from build123d import *

# Parameters (mm, degrees)
SKETCH1_R               = 9.525
BOSS_EXTRUDE1_DEPTH     = 25.4
CUT_EXTRUDE1_DEPTH      = 29.750847814
CUT_EXTRUDE1_DEPTH_BACK = 29.750847814
SKETCH2_R               = 3.175
SKETCH3_W               = 33.02
SKETCH3_H               = 34.544
BOSS_EXTRUDE2_DEPTH     = 254
BOSS_EXTRUDE3_DEPTH     = 22.225
SKETCH5_R               = 19.05
BOSS_EXTRUDE4_DEPTH     = 76.2
SKETCH6_W               = 19.05
SKETCH6_H               = 17.78
SKETCH6_R               = 3.175
BOSS_EXTRUDE5_DEPTH     = 8.89
FILLET1_R               = 2.54


with BuildPart() as part:
    # Sketch1 → Boss-Extrude1 (new body)
    with BuildSketch(Plane(origin=(0, 0, 0), x_dir=(0, 0, -1), z_dir=(1, 0, 0))):
        Circle(SKETCH1_R)
    extrude(amount=BOSS_EXTRUDE1_DEPTH)

    # Sketch2 → Cut-Extrude1 (cut, two sides: drawn at the far end of the back side and taken through both)
    with BuildSketch(Plane.XY.offset(-CUT_EXTRUDE1_DEPTH_BACK)):
        with Locations((15.24, 0)):
            Circle(SKETCH2_R)
    extrude(amount=CUT_EXTRUDE1_DEPTH + CUT_EXTRUDE1_DEPTH_BACK, mode=Mode.SUBTRACT)

    # Sketch3 → Boss-Extrude2 (add)
    with BuildSketch(Plane.ZY):
        Rectangle(SKETCH3_W, SKETCH3_H)
    extrude(amount=BOSS_EXTRUDE2_DEPTH)

    # Sketch4 → Boss-Extrude3 (add)
    with BuildSketch(Plane.ZY.offset(254)):
        with BuildLine():
            Line((-20.193, 17.272), (20.193, 17.272))
            Line((20.193, 17.272), (20.193, -38.735))
            ThreePointArc((20.193, -38.735), (0, -58.928), (-20.193, -38.735))
            Line((-20.193, -38.735), (-20.193, 17.272))
        make_face()
    extrude(amount=BOSS_EXTRUDE3_DEPTH)

    # Sketch5 → Boss-Extrude4 (add)
    with BuildSketch(Plane(origin=(-254, 0, 0), x_dir=(0, 0, -1), z_dir=(1, 0, 0))):
        with Locations(Location((0, -38.735, 0), (0, 0, 180))):
            Circle(SKETCH5_R)
    extrude(amount=BOSS_EXTRUDE4_DEPTH)

    # Sketch6 → Boss-Extrude5 (add, symmetric)
    with BuildSketch(Plane.XY):
        with Locations((-285.75, -1.778)):
            Rectangle(SKETCH6_W, SKETCH6_H)
        with Locations((-285.75, -1.778)):
            Circle(SKETCH6_R, mode=Mode.SUBTRACT)
    extrude(amount=BOSS_EXTRUDE5_DEPTH, both=True)

    # Fillet1
    fillet1_edges = [part.edges().sort_by_distance(p)[0] for p in [
        (-276.225, -1.778, 8.89),
        (-276.225, -1.778, -8.89),
        (-276.225, -10.668, 0),
        (-276.225, 7.112, 0),
        (-295.275, 7.112, 0),
        (-295.275, -10.668, 0),
    ]]
    fillet(fillet1_edges, radius=FILLET1_R)


solid = part.part
The model under review builds one solid part; all positions refer to its coordinate system, in mm. A direction names the side the tool comes from. Round coordinates to 2 decimals unless told otherwise and drop trailing zeros. Write each loop counter-clockwise with the first axis right and the second up, starting at its lowest first coordinate (ties: lowest second). Pieces come first, ordered by that corner, then holes. Notation, with made-up numbers: M -23,43 L 31,43 A18 cw 31,51 Z; hole C 87,31.25 d3. An arc over 180 degrees is marked long. Answer as CSV lines item,"result". Start each with the question number.
Q1. Consider section D-D, the plane x = -194.5. Give the boundary of the cut face in (y, z) (3 decimals), then the cut area to 3 significant figures.
Q2. Consider section B-B, the plane z = 0. Give the boundary of the cut face in (x, y) (3 decimals).
Q3. The part is to be moulded in two halves that separate along X. For faces 5 (the face through (-282.722, -0.824, -0.124)), 6 (the face through (-125, 0, -16.51)), 7 (the face through (0, 8, 7)), say which applies: +X half, -X half, draft (parallel to the pull), parting line (faces both ways), or undercut.
Q4. Wall thickness on line 1 along X through (y, z) = (0, -1.75) (3 decimals); line 2 along Y through (x, z) = (-248, 0) (3 decimals); line 3 along Y through (x, z) = (-285.75, 0.25): over which ranges is each line inside the solid? List them lowest first.
Q5. Tool access review of faces 1 (the face through (-286, 7.112, 0)), 2 (the face through (12.52, -3.65, -8.8)), 3 (the face through (-289, 0, 8.89)), 4 (the face through (-289, 0, -8.89)): name each direction out of +Z, -Z, +X, -X, +Y, -Y from which nothing blocks a thin tool from reaching the whole face with its end or side.
Q6. Clearance check with flat-ended pins moving along their axes: P1, Ø11.5, axis at y = -34, z = -7.5, coming from the +X side; P2, Ø1.5, axis at x = -7.5, z = 6.5, coming from the -Y side; P3, Ø11, axis at x = -286.5, z = 1.5, coming from the -Y side. State where each tip first meets the part, or that it passes through.
Q7. Consider section C-C, the plane y = -26. Give the boundary of the cut face in (x, z) (3 decimals).
Q8. Consider section A-A, the plane x = -285.75. Give the boundary of the cut face in (y, z).
Result set:
1,outline,"C -38.735,0 d38.1; M -17.272,-16.51 L 17.272,-16.51 L 17.272,16.51 L -17.272,16.51 Z"
1,area,"2,280 mm²"
2,outline,"M -295.275,-8.128 A2.54 ccw -292.735,-10.668 L -278.765,-10.668 A2.54 cw -276.225,-13.208 L -276.225,-58.928 L -254,-58.928 L -254,-57.785 L -177.8,-57.785 L -177.8,-19.685 L -254,-19.685 L -254,-17.272 L 0,-17.272 L 0,-9.525 L 25.4,-9.525 L 25.4,9.525 L 0,9.525 L 0,17.272 L -276.225,17.272 L -276.225,9.652 A2.54 cw -278.765,7.112 L -292.735,7.112 A2.54 ccw -295.275,4.572 Z; hole C -285.75,-1.778 d6.35; hole C 15.24,0 d6.35"
3,face 5,"undercut"
3,face 6,"draft"
3,face 7,"+X half"
4,line 1,"x = -295.275 to -288.38, -283.12 to 12.065, 18.415 to 25.4"
4,line 2,"y = -57.785 to -19.685, -17.272 to 17.272"
4,line 3,"y = -10.67 to -4.95, 1.4 to 7.11"
5,face 1,"+Z, -Z, -X, +Y"
5,face 2,"+X"
5,face 3,"+Z, -X, +Y, -Y"
5,face 4,"-Z, -X, +Y, -Y"
6,P1,"stops at x = -177.8"
6,P2,"stops at y = -17.27"
6,P3,"stops at y = -10.67"
7,outline,"M -276.225,-20.193 L -254,-20.193 L -254,-14.168 L -177.8,-14.168 L -177.8,14.168 L -254,14.168 L -254,20.193 L -276.225,20.193 Z"
8,outline,"M -10.67,-8.89 L -4.95,-8.89 L -4.95,8.89 L -10.67,8.89 Z; M 1.4,-8.89 L 7.11,-8.89 L 7.11,8.89 L 1.4,8.89 Z"
